Here's the drawing with two shaded views (mm, measured from the low corner). I have some questions. A direction names the side the tool comes from. Coordinates: 2 decimals unless noted, no trailing zeros. Loops run counter-clockwise (first coordinate to the right, second up) from the corner with the lowest first, then second, coordinate; pieces in that order, holes last. Notation, with made-up numbers: (15.5, 31.25) -> (48.5, 31.25) arc R8 cw to (48.5, 43.25) -> close; hole circle Ø5 at (68.25, 76). An arc over 180 degrees is marked (long way). Answer as a JSON object with one key per item and string values. Group by question number.
1) Which directions (+Z, -Z, +X, -X, +Y, -Y) give clear straight access to the entire face, cutting with the end or side of a thin tool? Please do the marked faces 1, 2 and 3.
2) I'm going to push flat-ended pins straight in: pin 1 (3 mm diameter, centred on y = 31.5, z = 88, fed in from +X); pin 2 (2 mm diameter, centred on x = 126.5, z = 38.5, fed in from +Y); pin 3 (12 mm diameter, centred on x = 62.5, y = 107, fed in from -Z). Where does each tip first touch, or does it pass through?
3) I need wall thicknesses on probe 1 along Z at (x, y) = (127, 23.5); probe 2 along Y at (x, z) = (90, 71); probe 3 along Y at (x, z) = (84.5, 87). Which ranges of each line are inside material? Lowest first, please. Write a range as [from, to].
4) I want a section at C-C (y = 78). Write out the boundary of the cut face in (x, z), then the cut area to 3 significant figures.
5) I want a section at A-A (z = 37.5). Write out the boundary of the cut face in (x, y).
6) I want a section at B-B (x = 75). Write out the boundary of the cut face in (y, z).
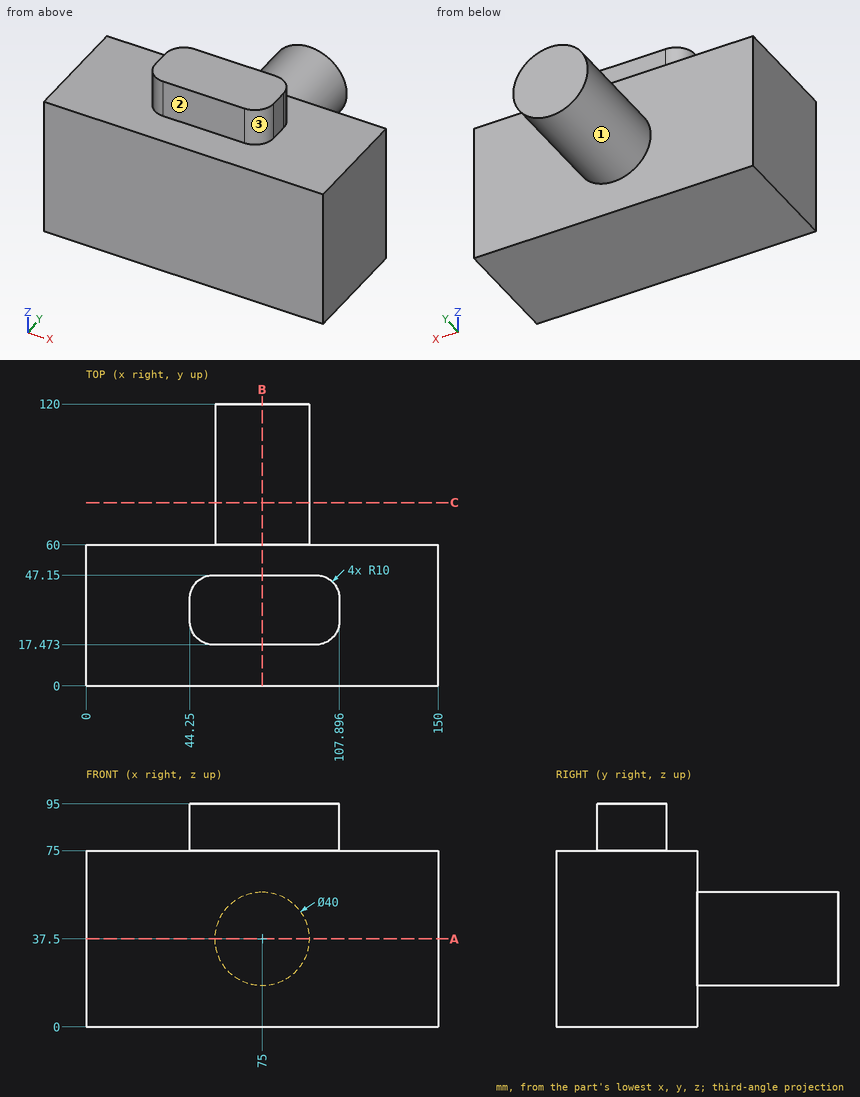
Determined:
{
 "1": {"face 1": "+Y", "face 2": "+Z, +X, -X, -Y", "face 3": "+Z, +X, -Y"},
 "2": {"pin 1": "x = 107.9", "pin 2": "y = 60", "pin 3": "z = 18.59"},
 "3": {"probe 1": "[0, 75]", "probe 2": "[0, 60]", "probe 3": "[17.47, 47.15]"},
 "4": {"outline": "circle Ø40 at (75, 37.5)", "area": "1,260 mm^2"},
 "5": {"outline": "(0, 0) -> (150, 0) -> (150, 60) -> (95, 60) -> (95, 120) -> (55, 120) -> (55, 60) -> (0, 60) -> close"},
 "6": {"outline": "(0, 0) -> (60, 0) -> (60, 17.5) -> (120, 17.5) -> (120, 57.5) -> (60, 57.5) -> (60, 75) -> (47.15, 75) -> (47.15, 95) -> (17.47, 95) -> (17.47, 75) -> (0, 75) -> close"}
}
